from build123d import *

# Parameters (mm, degrees)
F0_W     = 254
F0_H     = 234.95
F0_W_2   = 3.175
F0_H_2   = 361.95
F1_DEPTH = 374.65
F2_DEPTH = 6.35


# Not quite as in the source:
# - a feature names something its author has since deleted; it is built from what else it names


with BuildPart() as f1:
    # F0 (on Front) → F1 (new body)
    with BuildSketch(Plane.XZ):
        Polygon((-153.0927574873, 0), (224.7322425127, 0), (224.7322425127, 361.95), (177.1072425127, 361.95), (-153.0927574873, 361.95), align=None)
        with Locations((37.4072425127, 180.975)):
            Rectangle(F0_W, F0_H, mode=Mode.SUBTRACT)
        Polygon((231.0822425127, 361.95), (231.0822425127, 0), (608.9072425127, 0), (608.9072425127, 361.95), (278.7072425127, 361.95), align=None)
        with Locations((418.4072425127, 180.975)):
            Rectangle(F0_W, F0_H, mode=Mode.SUBTRACT)
        with Locations((37.4072425127, 180.975)):
            Rectangle(F0_W, F0_H)
        with Locations((418.4072425127, 180.975)):
            Rectangle(F0_W, F0_H)
        with Locations((226.3197425127, 180.975)):
            Rectangle(F0_W_2, F0_H_2)
        with Locations((229.4947425127, 180.975)):
            Rectangle(F0_W_2, F0_H_2)
    extrude(amount=-F1_DEPTH)

    # F0 (on Front) → F2 (cut)
    with BuildSketch(Plane.XZ):
        with Locations((226.3197425127, 180.975)):
            Rectangle(F0_W_2, F0_H_2)
        with Locations((229.4947425127, 180.975)):
            Rectangle(F0_W_2, F0_H_2)
        with Locations((37.4072425127, 180.975)):
            Rectangle(F0_W, F0_H)
        with Locations((418.4072425127, 180.975)):
            Rectangle(F0_W, F0_H)
    extrude(amount=-F2_DEPTH, mode=Mode.SUBTRACT)


solid = f1.part
Geometry: final body of the model. Coordinates: model frame, mm. Coordinates: 2 decimals unless noted, no trailing zeros.
(1) Material intervals for probe 1 along Y at (x, z) = (303, 75), sorted ascending.
(2) Draft query along Z for faces 1 (the face through (233, 185, 361.95)), 2 (the face through (36, 6.35, 183)), 3 (the face through (417, 0, 304)), 4 (the face through (417, 6.35, 183)). Return one class per face: pulls with the +Z half, pulls with the -Z half, needs draft (parallel to the pull), parting line crosses it, or undercut.
(3) First-contact query: pin 1 (3 mm diameter, centred on x = 228.5, z = 97, fed in from -Y). Flat tip, straight axial feed; report the tip coordinate or a pass-through.
Solution:
1. probe 1: y = 6.35 to 374.65
2. face 1: pulls with the +Z half
2. face 2: undercut
2. face 3: needs draft
2. face 4: undercut
3. pin 1: stops at y = 6.35
